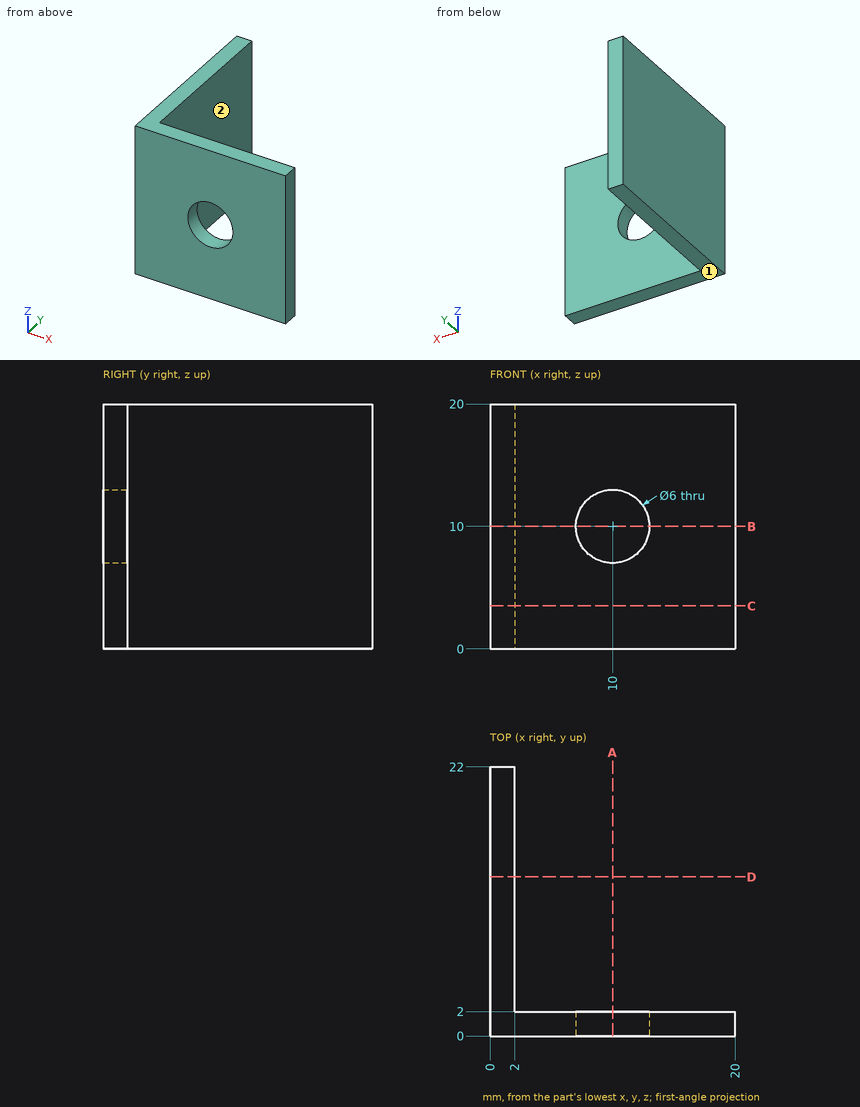
Geometry check sheet. Reference: drawing and pictorial views, mm from the part's lowest x, y, z. A direction names the side the tool comes from. Round coordinates to 2 decimals unless told otherwise and drop trailing zeros. Loops run counter-clockwise (first coordinate to the right, second up) from the corner with the lowest first, then second, coordinate; pieces in that order, holes last. Notation, with made-up numbers: (-4, -1) - (21, -1) arc R16 ccw to (21, 9) - close; hole circle Ø7 at (85, 42.25). An arc over 180 degrees is marked (long way). One line per question, with ' | ' between items. Start each with the question number.
1. Scan lines: line 1 (X direction, y = 1.25, z = 10); line 2 (X direction, y = 14.75, z = 10.75). Record each from-to range of solid material in increasing order. Write a range as [from, to].
2. Cross-section at A-A on x = 10. Record the cut outline in (y, z), then the cut area to 3 significant figures.
3. Cross-section at D-D on y = 13. Record the cut outline in (x, z), then the cut area to 3 significant figures.
4. Depth check by flat-ended pin: pin 1 (8 mm diameter, centred on x = 12, z = 15.5, fed in from +Y); pin 2 (6 mm diameter, centred on y = 13, z = 9.5, fed in from +X). Enter the tip coordinate at first touch or a pass-through.
5. Tool access check on the marked faces 1 and 2. Record the directions out of +Z, -Z, +X, -X, +Y, -Y that give a thin tool (end or side, any length) a straight path to the whole face; none if there is none.
6. Cross-section at C-C on z = 3.5. Record the cut outline in (x, y).
7. Cross-section at B-B on z = 10. Record the cut outline in (x, y).
Taken from the geometry:
1) line 1: [0, 7], [13, 20] | line 2: [0, 2]
2) outline: (0, 0) - (2, 0) - (2, 7) - (0, 7) - close; (0, 13) - (2, 13) - (2, 20) - (0, 20) - close | area: 28.0 mm²
3) outline: (0, 0) - (2, 0) - (2, 20) - (0, 20) - close | area: 40.0 mm²
4) pin 1: y = 2 | pin 2: x = 2
5) face 1: -Z, +X, -X, +Y, -Y | face 2: +Z, -Z, +X, +Y
6) outline: (0, 0) - (20, 0) - (20, 2) - (2, 2) - (2, 22) - (0, 22) - close
7) outline: (0, 0) - (7, 0) - (7, 2) - (2, 2) - (2, 22) - (0, 22) - close; (13, 0) - (20, 0) - (20, 2) - (13, 2) - close
